Could you check a few things on this model? Use its own coordinates, in mm. Face numbers are marked on the shaded views. A direction names the side the tool comes from. Give positions to 0.01 mm unless a question says otherwise; leave off trailing zeros. Loops run counter-clockwise (first coordinate to the right, second up) from the corner with the lowest first, then second, coordinate; pieces in that order, holes last. Notation, with made-up numbers: M 25.5,67 L 57.5,67 A13 ccw 57.5,90 Z; hole C -13,13.5 d1. An arc over 180 degrees is marked long. Use CSV: the item, a comma, the result in double quotes.
Autodesk Inventor part; units mm, degrees
ref_plane "YZ Plane" through (0, 0, 0) normal (1, 0, 0) x (0, 1, 0)
ref_plane "XZ Plane" through (0, 0, 0) normal (0, 1, 0) x (-1, 0, 0)
ref_plane "XY Plane" through (0, 0, 0) normal (0, 0, 1) x (1, 0, 0)
sketch "Esboço1" plane through (0, 0, 0) normal (0, 0, 1) x (1, 0, 0)
  line L0 (-7.5, 0) -> (-7.5, 3.25)
  line L1 (-7.5, 3.25) -> (-6.95, 3.25)
  line L2 (-6.95, 3.25) -> (-6.95, 4.35)
  line L3 (-6.95, 4.35) -> (-7.5, 4.35)
  line L4 (-7.5, 4.35) -> (-7.5, 19.65)
  line L5 (-7.5, 19.65) -> (-6.95, 19.65)
  line L6 (-6.95, 19.65) -> (-6.95, 20.75)
  line L7 (-6.95, 20.75) -> (-7.5, 20.75)
  line L8 (-7.5, 20.75) -> (-7.5, 24)
  line L9 (-7.5, 24) -> (-6.5, 24)
  line L10 (-7.5, 0) -> (-6.5, 0)
  line L11 (-6.5, 0) -> (0, 0) construction
  line L12 (0, 0) -> (0, 24) construction
  line L13 (0, 24) -> (-6.5, 24) construction
  line L14 (-6.5, 24) -> (-6.5, 0)
  dimension "d0" = 6.5
  dimension "d1" = 24
  dimension "d4" = 0.55
  dimension "d5" = 1.1
  dimension "d6" = 1.1
  dimension "d8" = 1
  dimension "d26" = 17.5
  dimension "d27" = 3.25
sketch "Esboço3" plane through (0, 0, 0) normal (0, 0, 1) x (1, 0, 0)
  line L0 (0, 24) -> (0, 0) construction
  line L1 (0, 24) -> (0, 35.5) construction
  line L2 (0, 0) -> (0, 1.5) construction
  line L3 (-4, 0) -> (-4, 24)
  line L4 (-4, 0) -> (-5, 0)
  line L5 (-5, 24) -> (-4, 24)
  line L6 (-5, 1.5) -> (-6.5, 1.5)
  line L7 (-6.5, 1.5) -> (-6.5, 22.5)
  line L8 (-6.5, 22.5) -> (-5, 22.5)
  line L9 (-5, 0) -> (-5, 1.5)
  line L10 (-5, 22.5) -> (-5, 24)
  dimension "d28" = 24
  dimension "d30" = 4
  dimension "d31" = 21
  dimension "d32" = 24
  dimension "d33" = 1.5
  dimension "d34" = 2.5
  dimension "d36" = 1
  dimension "d37" = 1
revolve "Revolução1" add sketch "Esboço3" angle 360 about axis through (0, 24, 0) along (0, -1, 0)
revolve "Revolução2" add sketch "Esboço1" angle 360 about axis through (0, 0, 0) along (0, 1, 0)
equation "\"d6\" = d5"
equation "\"d27\" = -0.5 * d26 + 0.5 * d1"
equation "\"d33\" = -0.5 * d31 + 0.5 * d32"
equation "\"d37\" = d36"
properties part number "rolamento_linear_lm8uu.iam"
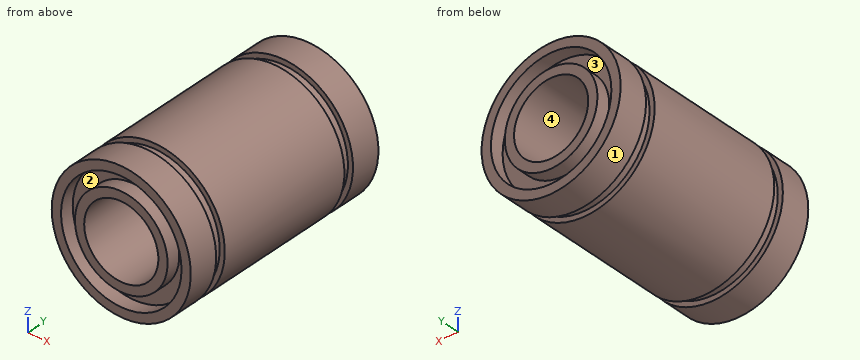
1. If we mould it in two halves opening along Z, with no side actions, what happens to the marked faces 1 and 2? For each: +Z half, -Z half, draft (parallel to the pull), parting line (faces both ways), or undercut.
Outcome:
face 1,"parting line"
face 2,"undercut"
2. I want a section at A-A, the plane y = 12.75. List the corners of the cut face in (x, z) for me.
Outcome:
outline,"C 0,0 d15; hole C 0,0 d8"
3. I want a section at B-B, the plane x = -6. List the corners of the cut face in (y, z) for me.
Outcome:
outline,"M 0,-4.5 L 3.25,-4.5 L 3.25,-3.51 L 4.35,-3.51 L 4.35,-4.5 L 19.65,-4.5 L 19.65,-3.51 L 20.75,-3.51 L 20.75,-4.5 L 24,-4.5 L 24,-2.5 L 22.5,-2.5 L 22.5,2.5 L 24,2.5 L 24,4.5 L 20.75,4.5 L 20.75,3.51 L 19.65,3.51 L 19.65,4.5 L 4.35,4.5 L 4.35,3.51 L 3.25,3.51 L 3.25,4.5 L 0,4.5 L 0,2.5 L 1.5,2.5 L 1.5,-2.5 L 0,-2.5 Z"
4. Which directions (+Z, -Z, +X, -X, +Y, -Y) give clear straight access to the entire face, cutting with the end or side of a thin tool? Please do the marked faces 3 and 4.
Outcome:
face 3,"+Y"
face 4,"+Y, -Y"
5. I'm going to push flat-ended pins straight in: pin 1 Ø1.5 at (y, z) = (14, 1.5) entering from +X; pin 2 Ø1 at (x, y) = (2, 14.5) entering from -Z. Where does each tip first touch, or does it pass through?
Outcome:
pin 1,"x = 7.46"
pin 2,"z = -7.35"
6. Please list where these lines run through material, in increasing order: line 1 (Y direction, x = 4.75, z = -5.25); line 2 (Z direction, x = 0, y = 22.9); line 3 (Z direction, x = 0, y = 8.25).
Outcome:
line 1,"0 to 3.25, 4.35 to 19.65, 20.75 to 24"
line 2,"-7.5 to -6.5, -5 to -4, 4 to 5, 6.5 to 7.5"
line 3,"-7.5 to -4, 4 to 7.5"
